Part model, mm, in its own coordinate system. A direction names the side the tool comes from. Give positions to 0.01 mm unless a question says otherwise; leave off trailing zeros. One line per item, written item: value.
```python
from build123d import *

# Parameters (mm, degrees)
SKETCH3_R          = 2.5
CUT_EXTRUDE1_DEPTH = 4
SKETCH6_R          = 3
CUT_EXTRUDE4_DEPTH = 11
SKETCH7_R          = 3.3
CUT_EXTRUDE5_DEPTH = 10
SKETCH9_R          = 1
CUT_EXTRUDE7_DEPTH = 2
CUT_EXTRUDE8_REACH = 117.07
SKETCH10_R         = 3.3
CHAMFER1_SIZE      = 0.5


with BuildPart() as part:
    # Sketch2 → Revolve1 (revolve)
    with BuildSketch(Plane.XY, mode=Mode.PRIVATE) as revolve1_sk:
        Polygon((0, 80), (0, 52.5), (11, 52.5), (11, 32.5), (18, 32.5), (18, 29.5), (21, 29.5), (21, 80), align=None)
    revolve(revolve1_sk.sketch.rotate(Axis((0, 0, 0), (1, 0, 0)), 90), axis=Axis((0, 0, 0), (1, 0, 0)))

    # Sketch3 → Cut-Extrude1 (cut)
    with BuildSketch(Plane.ZY):
        with Locations((0, 60)):
            Circle(SKETCH3_R)
        with Locations((12.077911205, 58.771796475)):
            Circle(SKETCH3_R)
        with Locations((23.661351307, 55.137468697)):
            Circle(SKETCH3_R)
        with Locations((34.276092906, 49.245806472)):
            Circle(SKETCH3_R)
        with Locations((43.487567234, 41.338015145)):
            Circle(SKETCH3_R)
        with Locations((50.91865545, 31.73784062)):
            Circle(SKETCH3_R)
        with Locations((56.265127929, 20.838315171)):
            Circle(SKETCH3_R)
        with Locations((59.30809946, 9.08566665)):
            Circle(SKETCH3_R)
        with Locations((59.92299043, -3.03895013)):
            Circle(SKETCH3_R)
        with Locations((58.084627132, -15.039151936)):
            Circle(SKETCH3_R)
        with Locations((53.868272374, -26.423649093)):
            Circle(SKETCH3_R)
        with Locations((47.446544216, -36.726358953)):
            Circle(SKETCH3_R)
        with Locations((39.082348963, -45.525487362)):
            Circle(SKETCH3_R)
        with Locations((29.118117752, -52.460796969)):
            Circle(SKETCH3_R)
        with Locations((17.961787378, -57.248355384)):
            Circle(SKETCH3_R)
        with Locations((6.070099319, -59.692159404)):
            Circle(SKETCH3_R)
        with Locations((-6.070099319, -59.692159404)):
            Circle(SKETCH3_R)
        with Locations((-17.961787378, -57.248355384)):
            Circle(SKETCH3_R)
        with Locations((-29.118117752, -52.460796969)):
            Circle(SKETCH3_R)
        with Locations((-39.082348963, -45.525487362)):
            Circle(SKETCH3_R)
        with Locations((-47.446544216, -36.726358953)):
            Circle(SKETCH3_R)
        with Locations((-53.868272374, -26.423649093)):
            Circle(SKETCH3_R)
        with Locations((-58.084627132, -15.039151936)):
            Circle(SKETCH3_R)
        with Locations((-59.92299043, -3.03895013)):
            Circle(SKETCH3_R)
        with Locations((-59.30809946, 9.08566665)):
            Circle(SKETCH3_R)
        with Locations((-56.265127929, 20.838315171)):
            Circle(SKETCH3_R)
        with Locations((-50.91865545, 31.73784062)):
            Circle(SKETCH3_R)
        with Locations((-43.487567234, 41.338015145)):
            Circle(SKETCH3_R)
        with Locations((-34.276092906, 49.245806472)):
            Circle(SKETCH3_R)
        with Locations((-23.661351307, 55.137468697)):
            Circle(SKETCH3_R)
        with Locations((-12.077911205, 58.771796475)):
            Circle(SKETCH3_R)
    extrude(amount=-CUT_EXTRUDE1_DEPTH, mode=Mode.SUBTRACT)

    # Sketch6 → Cut-Extrude4 (cut)
    with BuildSketch(Plane.ZY):
        with Locations((53.875586653, 44.692517973)):
            Circle(SKETCH6_R)
        with Locations((69.69817519, -6.493410136)):
            Circle(SKETCH6_R)
        with Locations((44.692517973, -53.875586653)):
            Circle(SKETCH6_R)
        with Locations((-6.493410136, -69.69817519)):
            Circle(SKETCH6_R)
        with Locations((-53.875586653, -44.692517973)):
            Circle(SKETCH6_R)
        with Locations((-69.69817519, 6.493410136)):
            Circle(SKETCH6_R)
        with Locations((-44.692517973, 53.875586653)):
            Circle(SKETCH6_R)
        with Locations((6.493410136, 69.69817519)):
            Circle(SKETCH6_R)
    extrude(amount=-CUT_EXTRUDE4_DEPTH, mode=Mode.SUBTRACT)

    # Sketch7 → Cut-Extrude5 (cut)
    with BuildSketch(Plane.ZY.offset(-21)):
        with Locations((53.875586653, 44.692517973)):
            Circle(SKETCH7_R)
        with Locations((69.69817519, -6.493410136)):
            Circle(SKETCH7_R)
        with Locations((44.692517973, -53.875586653)):
            Circle(SKETCH7_R)
        with Locations((-6.493410136, -69.69817519)):
            Circle(SKETCH7_R)
        with Locations((-53.875586653, -44.692517973)):
            Circle(SKETCH7_R)
        with Locations((-69.69817519, 6.493410136)):
            Circle(SKETCH7_R)
        with Locations((-44.692517973, 53.875586653)):
            Circle(SKETCH7_R)
        with Locations((6.493410136, 69.69817519)):
            Circle(SKETCH7_R)
    extrude(amount=CUT_EXTRUDE5_DEPTH, mode=Mode.SUBTRACT)

    # Sketch9 → Cut-Extrude7 (cut)
    with BuildSketch(Plane.ZY):
        with Locations((2.51770285, -71.46627686)):
            Circle(SKETCH9_R)
    extrude(amount=-CUT_EXTRUDE7_DEPTH, mode=Mode.SUBTRACT)

    # Sketch10 → Cut-Extrude8 (cut, up to next)
    with BuildSketch(Plane(origin=(21, 0, 0), x_dir=(0, 0, -1), z_dir=(1, 0, 0)), mode=Mode.PRIVATE) as cut_extrude8_sk1:
        with Locations((23.431880753, 37.241736861)):
            Circle(SKETCH10_R)
    cut_extrude8_tool1 = extrude(cut_extrude8_sk1.sketch, amount=-CUT_EXTRUDE8_REACH, mode=Mode.PRIVATE) & part.part
    # Sketch10 → Cut-Extrude8 (cut, up to next)
    with BuildSketch(Plane(origin=(21, 0, 0), x_dir=(0, 0, -1), z_dir=(1, 0, 0)), mode=Mode.PRIVATE) as cut_extrude8_sk2:
        with Locations((20.536349826, -38.913472421)):
            Circle(SKETCH10_R)
    cut_extrude8_tool2 = extrude(cut_extrude8_sk2.sketch, amount=-CUT_EXTRUDE8_REACH, mode=Mode.PRIVATE) & part.part
    # Sketch10 → Cut-Extrude8 (cut, up to next)
    with BuildSketch(Plane(origin=(21, 0, 0), x_dir=(0, 0, -1), z_dir=(1, 0, 0)), mode=Mode.PRIVATE) as cut_extrude8_sk3:
        with Locations((-43.968230579, 1.67173556)):
            Circle(SKETCH10_R)
    cut_extrude8_tool3 = extrude(cut_extrude8_sk3.sketch, amount=-CUT_EXTRUDE8_REACH, mode=Mode.PRIVATE) & part.part
    # Sketch10 → Cut-Extrude8 (cut, up to next)
    with BuildSketch(Plane(origin=(21, 0, 0), x_dir=(0, 0, -1), z_dir=(1, 0, 0)), mode=Mode.PRIVATE) as cut_extrude8_sk4:
        with Locations((-23.431880753, -37.241736861)):
            Circle(SKETCH10_R)
    cut_extrude8_tool4 = extrude(cut_extrude8_sk4.sketch, amount=-CUT_EXTRUDE8_REACH, mode=Mode.PRIVATE) & part.part
    # Sketch10 → Cut-Extrude8 (cut, up to next)
    with BuildSketch(Plane(origin=(21, 0, 0), x_dir=(0, 0, -1), z_dir=(1, 0, 0)), mode=Mode.PRIVATE) as cut_extrude8_sk5:
        with Locations((43.968230579, -1.67173556)):
            Circle(SKETCH10_R)
    cut_extrude8_tool5 = extrude(cut_extrude8_sk5.sketch, amount=-CUT_EXTRUDE8_REACH, mode=Mode.PRIVATE) & part.part
    add(cut_extrude8_tool1.solids().sort_by_distance((21, 37.241737, -23.431881))[0], mode=Mode.SUBTRACT)
    add(cut_extrude8_tool2.solids().sort_by_distance((21, -38.913472, -20.53635))[0], mode=Mode.SUBTRACT)
    add(cut_extrude8_tool3.solids().sort_by_distance((21, 1.671736, 43.968231))[0], mode=Mode.SUBTRACT)
    add(cut_extrude8_tool4.solids().sort_by_distance((21, -37.241737, 23.431881))[0], mode=Mode.SUBTRACT)
    add(cut_extrude8_tool5.solids().sort_by_distance((21, -1.671736, -43.968231))[0], mode=Mode.SUBTRACT)

    # Chamfer1
    chamfer1_edges = [part.edges().sort_by_distance(p)[0] for p in [
        (21, 53.875586653, -47.992517973),
        (21, -6.493410136, 66.39817519),
        (21, -53.875586653, 41.392517973),
        (21, -69.69817519, -9.793410136),
        (21, -44.692517973, -57.175586653),
        (21, 6.493410136, -72.99817519),
        (21, 69.69817519, 3.193410136),
        (21, 44.692517973, 50.575586653),
        (21, 37.241736861, -20.131880753),
        (21, -1.67173556, -40.668230579),
        (21, -38.913472421, -17.236349826),
        (21, 1.67173556, 47.268230579),
        (21, -37.241736861, 26.731880753),
    ]]
    chamfer(chamfer1_edges, length=CHAMFER1_SIZE)


solid = part.part
```
1) Which spindle directions (+Z, -Z, +X, -X, +Y, -Y) get a long thin tool onto all of the face, cutting with end or side? Do faces 1 (the face through (1.972, 43.817, 43.162)), 2 (the face through (15.82, -45.96, -50.83)), 3 (the face through (15.817, -0.681, -47.116)). Say none if no direction does.
Answer:
face 1: -X
face 2: +X
face 3: +X, -X
2) Wall check: line 1 along Z through (x, y) = (14, 4); line 2 along Z through (x, y) = (8, 8.5); line 3 along Y through (x, z) = (12, -21.5). Give the ranges that are in metal, low to high. Write a range as [from, to].
Answer:
line 1: z = [-79.9, -71.86], [-67.54, -32.25], [32.25, 41.63], [46.31, 79.9]
line 2: z = [-79.55, -71.93], [-67.47, -51.81], [51.81, 79.55]
line 3: y = [-77.06, -42.07], [-35.76, -24.37], [24.37, 34.57], [39.92, 77.06]
3) Drop flat-ended pins along their axis: P1, Ø1, axis at x = 2.5, y = -5.5, coming from the -Z side; P2, Ø5, axis at x = 7, y = -51.5, coming from the +Z side; P3, Ø5, axis at x = 8.5, z = 17.5, coming from the +Y side. Give the stop position or say it passes through.
Answer:
P1: stops at z = -79.84
P2: stops at z = 63.24
P3: stops at y = 78.58
4) Slice it at A-A on x = 7.5. Count the separate pieces of the cut face and the enclosed holes in it, then the cut area to 3 significant figures.
Answer:
separate pieces: 1
enclosed holes: 9
area: 11,200 mm2
